Design review of the part built by this model. Coordinates are the model's own, in mm. Face numbers are marked on the shaded views. A direction names the side the tool comes from. Coordinates: 2 decimals unless noted, no trailing zeros. Order: outer loops, then holes, each group sorted by start corner. A loop starts at its lowest first (then second) coordinate and runs counter-clockwise, first axis right, second up.
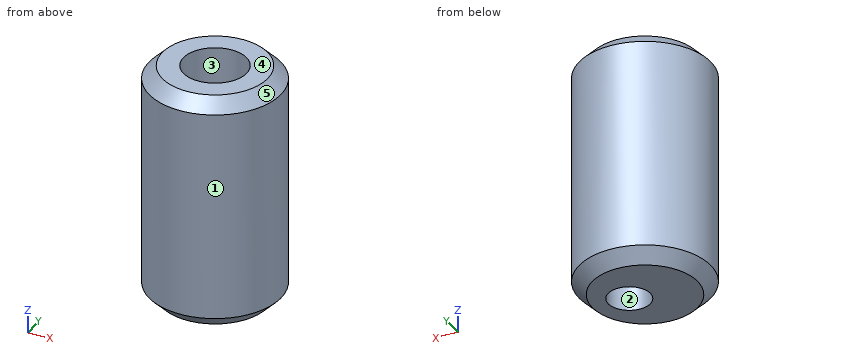
from build123d import *

# Parameters (mm, degrees)
F0_R     = 5
F1_DEPTH = 18
F2_R     = 2.4
F3_DEPTH = 12
F4_R     = 1.6
F5_DEPTH = 5
F6_SIZE  = 0.6
F7_SIZE  = 1


with BuildPart() as f1:
    # F0 (on Top) → F1 (new body)
    with BuildSketch(Plane.XY):
        Circle(F0_R)
    extrude(amount=F1_DEPTH)

    # F2 (on face) → F3 (cut)
    with BuildSketch(Plane.XY.offset(18)):
        Circle(F2_R)
    extrude(amount=-F3_DEPTH, mode=Mode.SUBTRACT)

    # F4 (on face) → F5 (cut)
    with BuildSketch(Plane(origin=(0, 0, 0), x_dir=(1, 0, 0), z_dir=(0, 0, -1))):
        with Locations((1.2, 0)):
            Circle(F4_R)
    extrude(amount=-F5_DEPTH, mode=Mode.SUBTRACT)

    # F6
    f6_edges = [f1.edges().sort_by_distance(p)[0] for p in [
        (-0.4, 0, 5),
        (-2.4, 0, 6),
    ]]
    chamfer(f6_edges, length=F6_SIZE)

    # F7
    f7_edges = [f1.edges().sort_by_distance(p)[0] for p in [
        (-5, 0, 0),
        (-5, 0, 18),
    ]]
    chamfer(f7_edges, length=F7_SIZE)


solid = f1.part
1. To check wall thickness, follow line 1 (Y direction, x = 1.2, z = 3.3); line 2 (Y direction, x = -1.75, z = 6.75); line 3 (X direction, y = -1, z = 2). State the ranges of each line that lie inside material, in increasing order.
2. Add section B-B (z = 12.75). Give the boundary of the cut face in (x, y).
3. Add section C-C (z = 5.5). Give the boundary of the cut face in (x, y).
4. For the marked faces 1 and 2, list the 3-axis set-ups (+Z, -Z, +X, -X, +Y, -Y) from which the entire face can be reached by the end or side of a thin tool; tool diameter is ignored.
5. Mouldability with a two-part tool opening along Y and no side actions: class the marked faces 3, 4 and 5 as pulls with the +Y half, pulls with the -Y half, needs draft (parallel to the pull), parting line crosses it, or undercut.
6. Insertion check: pin 1 (1.5 mm diameter, centred on x = 0, y = 3, fed in from -Z); pin 2 (2 mm diameter, centred on x = 1.5, y = 0, fed in from -Z); pin 3 (2 mm diameter, centred on y = -2.5, z = 14.5, fed in from -X); pin 4 (1.1 mm diameter, centred on x = -0.5, y = -1, fed in from +Z). Each pin has a flat end and moves straight along its axis. Give the tip position at first contact, or say it passes through.
7. Add section A-A (y = 0). Give the boundary of the cut face in (x, z).
Solution:
1. line 1: y = -4.85 to -1.6, 1.6 to 4.85
1. line 2: y = -4.68 to -1.64, 1.64 to 4.68
1. line 3: x = -4.9 to -0.05, 2.45 to 4.9
2. outline: circle Ø10 at (0, 0); hole circle Ø4.8 at (0, 0)
3. outline: circle Ø10 at (0, 0)
4. face 1: +Z, -Z
4. face 2: -Z
5. face 3: undercut
5. face 4: needs draft
5. face 5: parting line crosses it
6. pin 1: stops at z = 0
6. pin 2: stops at z = 4.7
6. pin 3: stops at x = -4.77
6. pin 4: stops at z = 6
7. outline: (-5, 1) - (-4, 0) - (-0.4, 0) - (-0.4, 4.4) - (0.2, 5) - (2.2, 5) - (2.8, 4.4) - (2.8, 0) - (4, 0) - (5, 1) - (5, 17) - (4, 18) - (2.4, 18) - (2.4, 6.6) - (1.8, 6) - (-1.8, 6) - (-2.4, 6.6) - (-2.4, 18) - (-4, 18) - (-5, 17) - close
